```python
from build123d import *

# Parameters (mm, degrees)
CYLINDER001_R     = 9.525
CYLINDER001_DEPTH = 254
CYLINDER_R        = 13.335
CYLINDER_DEPTH    = 254


with BuildPart() as f_0_75_id:
    # Cylinder001 → Cylinder001 (new body)
    with BuildSketch(Plane.XY):
        Circle(CYLINDER001_R)
    extrude(amount=CYLINDER001_DEPTH)


with BuildPart() as f_0_75in_x_10in_npt_pipe:
    # Cylinder → Cylinder (new body)
    with BuildSketch(Plane.XY):
        Circle(CYLINDER_R)
    extrude(amount=CYLINDER_DEPTH)

    # Cut: cut 0.75 ID
    add(f_0_75_id.part, mode=Mode.SUBTRACT)


solid = f_0_75in_x_10in_npt_pipe.part
```
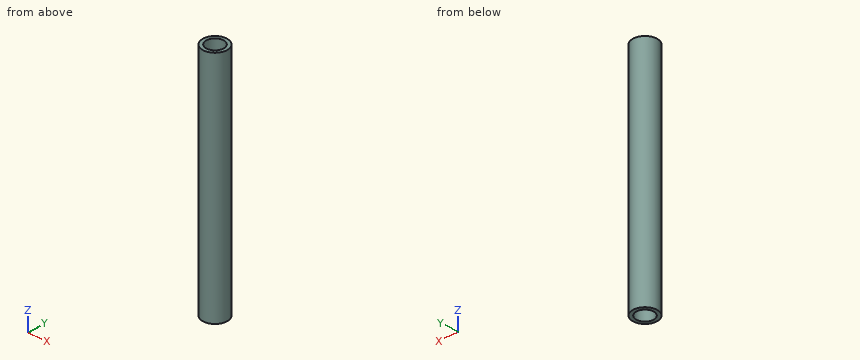
For this review, take the finished solid that the model builds, in its own axes (mm). Coordinates: 2 decimals unless noted, no trailing zeros. Write each loop counter-clockwise with the first axis right and the second up, starting at its lowest first coordinate (ties: lowest second). Pieces come first, ordered by that corner, then holes.
(1) Add section C-C on z = 232.5. Give the boundary of the cut face in (x, y) (3 decimals), then the cut area to 3 significant figures.
(2) Wall thickness on probe 1 along Y at (x, z) = (0, 183.5) (3 decimals); probe 2 along X at (y, z) = (0.5, 204); probe 3 along X at (y, z) = (-6, 33): over which ranges is each line inside the solid? List them lowest first.
(3) Add section A-A on y = 0. Give the boundary of the cut face in (x, z) (3 decimals), then the cut area to 3 significant figures.
(4) For pin 1 Ø1.5 at (x, z) = (-3, 164) entering from -Y; pin 2 Ø4 at (x, z) = (5, 127.5) entering from -Y; pin 3 Ø3 at (x, z) = (10, 102.5) entering from +Y, all flat-tipped, find the tip position at first contact; note any pin that passes through.
Answer sheet:
1. outline: circle Ø26.67 at (0, 0); hole circle Ø19.05 at (0, 0)
1. area: 274 mm2
2. probe 1: y = -13.335 to -9.525, 9.525 to 13.335
2. probe 2: x = -13.33 to -9.51, 9.51 to 13.33
2. probe 3: x = -11.91 to -7.4, 7.4 to 11.91
3. outline: (-13.335, 0) - (-9.525, 0) - (-9.525, 254) - (-13.335, 254) - close; (9.525, 0) - (13.335, 0) - (13.335, 254) - (9.525, 254) - close
3. area: 1,940 mm2
4. pin 1: stops at y = -13.14
4. pin 2: stops at y = -12.99
4. pin 3: stops at y = 10.27
